Geometry check sheet. Reference: the model listing, model coordinates, mm. A direction names the side the tool comes from. Coordinates: 2 decimals unless noted, no trailing zeros. Order: outer loops, then holes, each group sorted by start corner. A loop starts at its lowest first (then second) coordinate and runs counter-clockwise, first axis right, second up. Notation, with made-up numbers: (-21.5, 58) - (1.5, 58) arc R28 cw to (1.5, 97) - close; hole circle Ø5 at (-11.5, 17.5). An arc over 180 degrees is marked (long way). Put each result on its own line as item: value.
from build123d import *

# Parameters (mm, degrees)
CROQUIS1_W                         = 500
CROQUIS1_H                         = 510
SALIENTE_EXTRUIR1_DEPTH            = 6.35
CORTAR_EXTRUIR1_DEPTH              = 358.16287951
CORTAR_EXTRUIR2_DEPTH              = 358.16287951
TALADRO_ROSCADO_M6X1_01_AT_2_COUNT = 2
TALADRO_ROSCADO_M6X1_01_AT_2_PITCH = 44
TALADRO_ROSCADO_M6X1_01_AT_3_COUNT = 2
TALADRO_ROSCADO_M6X1_01_AT_3_PITCH = 71.217975259
TALADRO_ROSCADO_M6X1_01_AT_4_COUNT = 2
TALADRO_ROSCADO_M6X1_01_AT_4_PITCH = 56
MATRIZL1_COUNT                     = 4
MATRIZL1_PITCH                     = 10
TALADRO_ROSCADO_M5X0_82_D          = 4.2
TALADRO_ROSCADO_M6X1_02_D          = 5


with BuildPart() as part:
    # Croquis1 → Saliente-Extruir1 (new body)
    with BuildSketch(Plane.XY):
        Rectangle(CROQUIS1_W, CROQUIS1_H)
    extrude(amount=SALIENTE_EXTRUIR1_DEPTH)

    # Croquis2 → Cortar-Extruir1 (cut, through all)
    with BuildSketch(Plane.XY.offset(6.35)):
        with BuildLine():
            Line((-211, -225.15), (-131, -225.15))
            ThreePointArc((-131, -225.15), (-124.65, -231.5), (-131, -237.85))
            Line((-131, -237.85), (-211, -237.85))
            ThreePointArc((-211, -237.85), (-217.35, -231.5), (-211, -225.15))
        make_face()
        with BuildLine():
            Line((-211, 237.85), (-131, 237.85))
            ThreePointArc((-131, 237.85), (-124.65, 231.5), (-131, 225.15))
            Line((-131, 225.15), (-211, 225.15))
            ThreePointArc((-211, 225.15), (-217.35, 231.5), (-211, 237.85))
        make_face()
        with BuildLine():
            Line((131, 237.85), (211, 237.85))
            ThreePointArc((211, 237.85), (217.35, 231.5), (211, 225.15))
            Line((211, 225.15), (131, 225.15))
            ThreePointArc((131, 225.15), (124.65, 231.5), (131, 237.85))
        make_face()
        with BuildLine():
            Line((131, -225.15), (211, -225.15))
            ThreePointArc((211, -225.15), (217.35, -231.5), (211, -237.85))
            Line((211, -237.85), (131, -237.85))
            ThreePointArc((131, -237.85), (124.65, -231.5), (131, -225.15))
        make_face()
        with BuildLine():
            Line((-14.65, -160.73303664), (-14.65, -182.26696336))
            ThreePointArc((-14.65, -182.26696336), (-21, -184), (-27.35, -182.26696336))
            Line((-27.35, -182.26696336), (-27.35, -160.73303664))
            ThreePointArc((-27.35, -160.73303664), (-21, -159), (-14.65, -160.73303664))
        make_face()
    extrude(amount=-CORTAR_EXTRUIR1_DEPTH, mode=Mode.SUBTRACT)

    # Croquis4 → Cortar-Extruir2 (cut, through all)
    with BuildSketch(Plane.XY.offset(6.35)):
        with BuildLine():
            Line((-150, 130), (150, 130))
            ThreePointArc((150, 130), (175, 105), (150, 80))
            Line((150, 80), (-150, 80))
            ThreePointArc((-150, 80), (-175, 105), (-150, 130))
        make_face()
        with BuildLine():
            Line((-150, -28.46), (150, -28.46))
            ThreePointArc((150, -28.46), (175, -53.46), (150, -78.46))
            Line((150, -78.46), (-150, -78.46))
            ThreePointArc((-150, -78.46), (-175, -53.46), (-150, -28.46))
        make_face()
    extrude(amount=-CORTAR_EXTRUIR2_DEPTH, mode=Mode.SUBTRACT)

    # Croquis7 → Taladro roscado M6x1.01 (revolve, cut)
    with BuildSketch(Plane(origin=(-242, 217, 6.35), x_dir=(0, -1, 0), z_dir=(1, 0, 0))):
        Polygon((0, 0), (0, 18.502151548), (2.5, 17), (2.5, 0), align=None)
    taladro_roscado_m6x1_01 = revolve(axis=Axis((-242, 217, 12.7), (0, 0, -1)), mode=Mode.SUBTRACT)

    # Taladro roscado M6x1.01 at 2: Taladro roscado M6x1.01 ×2
    with Locations(*[(i * TALADRO_ROSCADO_M6X1_01_AT_2_PITCH, 0, 0) for i in range(1, TALADRO_ROSCADO_M6X1_01_AT_2_COUNT)]):
        add(taladro_roscado_m6x1_01, mode=Mode.SUBTRACT)

    # Taladro roscado M6x1.01 at 3: Taladro roscado M6x1.01 ×2
    with Locations(*[Vector(0.6178215519319036, -0.7863183388224226, 0) * (i * TALADRO_ROSCADO_M6X1_01_AT_3_PITCH) for i in range(1, TALADRO_ROSCADO_M6X1_01_AT_3_COUNT)]):
        add(taladro_roscado_m6x1_01, mode=Mode.SUBTRACT)

    # Taladro roscado M6x1.01 at 4: Taladro roscado M6x1.01 ×2
    with Locations(*[(0, -i * TALADRO_ROSCADO_M6X1_01_AT_4_PITCH, 0) for i in range(1, TALADRO_ROSCADO_M6X1_01_AT_4_COUNT)]):
        add(taladro_roscado_m6x1_01, mode=Mode.SUBTRACT)

    # MatrizL1: Taladro roscado M6x1.01 ×4
    with Locations(*[(0, -i * MATRIZL1_PITCH, 0) for i in range(1, MATRIZL1_COUNT)]):
        add(taladro_roscado_m6x1_01, mode=Mode.SUBTRACT)

    # MatrizL1 copy 1 sketch → MatrizL1 copy 1 (revolve, cut)
    with BuildSketch(Plane(origin=(-198, 207, 6.35), x_dir=(0, -1, 0), z_dir=(1, 0, 0))):
        Polygon((0, 0), (0, 18.502151548), (2.5, 17), (2.5, 0), align=None)
    revolve(axis=Axis((-198, 207, 12.7), (0, 0, -1)), mode=Mode.SUBTRACT)

    # MatrizL1 copy 2 sketch → MatrizL1 copy 2 (revolve, cut)
    with BuildSketch(Plane(origin=(-198, 197, 6.35), x_dir=(0, -1, 0), z_dir=(1, 0, 0))):
        Polygon((0, 0), (0, 18.502151548), (2.5, 17), (2.5, 0), align=None)
    revolve(axis=Axis((-198, 197, 12.7), (0, 0, -1)), mode=Mode.SUBTRACT)

    # MatrizL1 copy 3 sketch → MatrizL1 copy 3 (revolve, cut)
    with BuildSketch(Plane(origin=(-198, 187, 6.35), x_dir=(0, -1, 0), z_dir=(1, 0, 0))):
        Polygon((0, 0), (0, 18.502151548), (2.5, 17), (2.5, 0), align=None)
    revolve(axis=Axis((-198, 187, 12.7), (0, 0, -1)), mode=Mode.SUBTRACT)

    # MatrizL1 copy 4 sketch → MatrizL1 copy 4 (revolve, cut)
    with BuildSketch(Plane(origin=(-198, 151, 6.35), x_dir=(0, -1, 0), z_dir=(1, 0, 0))):
        Polygon((0, 0), (0, 18.502151548), (2.5, 17), (2.5, 0), align=None)
    revolve(axis=Axis((-198, 151, 12.7), (0, 0, -1)), mode=Mode.SUBTRACT)

    # MatrizL1 copy 5 sketch → MatrizL1 copy 5 (revolve, cut)
    with BuildSketch(Plane(origin=(-198, 141, 6.35), x_dir=(0, -1, 0), z_dir=(1, 0, 0))):
        Polygon((0, 0), (0, 18.502151548), (2.5, 17), (2.5, 0), align=None)
    revolve(axis=Axis((-198, 141, 12.7), (0, 0, -1)), mode=Mode.SUBTRACT)

    # MatrizL1 copy 6 sketch → MatrizL1 copy 6 (revolve, cut)
    with BuildSketch(Plane(origin=(-198, 131, 6.35), x_dir=(0, -1, 0), z_dir=(1, 0, 0))):
        Polygon((0, 0), (0, 18.502151548), (2.5, 17), (2.5, 0), align=None)
    revolve(axis=Axis((-198, 131, 12.7), (0, 0, -1)), mode=Mode.SUBTRACT)

    # MatrizL1 copy 7 sketch → MatrizL1 copy 7 (revolve, cut)
    with BuildSketch(Plane(origin=(-242, 151, 6.35), x_dir=(0, -1, 0), z_dir=(1, 0, 0))):
        Polygon((0, 0), (0, 18.502151548), (2.5, 17), (2.5, 0), align=None)
    revolve(axis=Axis((-242, 151, 12.7), (0, 0, -1)), mode=Mode.SUBTRACT)

    # MatrizL1 copy 8 sketch → MatrizL1 copy 8 (revolve, cut)
    with BuildSketch(Plane(origin=(-242, 141, 6.35), x_dir=(0, -1, 0), z_dir=(1, 0, 0))):
        Polygon((0, 0), (0, 18.502151548), (2.5, 17), (2.5, 0), align=None)
    revolve(axis=Axis((-242, 141, 12.7), (0, 0, -1)), mode=Mode.SUBTRACT)

    # MatrizL1 copy 9 sketch → MatrizL1 copy 9 (revolve, cut)
    with BuildSketch(Plane(origin=(-242, 131, 6.35), x_dir=(0, -1, 0), z_dir=(1, 0, 0))):
        Polygon((0, 0), (0, 18.502151548), (2.5, 17), (2.5, 0), align=None)
    revolve(axis=Axis((-242, 131, 12.7), (0, 0, -1)), mode=Mode.SUBTRACT)

    # Taladro roscado M5x0.82 (through all)
    with Locations(Plane.XY.offset(6.35)):
        with Locations((-125, 193.27), (-125, 163.27), (25, 193.27), (25, 163.27), (175, 193.27), (175, 163.27), (175, -111.73), (175, -141.73), (25, -111.73), (25, -141.73), (-125, -111.73), (-125, -141.73)):
            Hole(TALADRO_ROSCADO_M5X0_82_D / 2)

    # Taladro roscado M6x1.02 (through all)
    with Locations(Plane.XY.offset(6.35)):
        with Locations((-229.542734314, 48.77), (-216.542734314, 48.77), (-216.542734314, 2.77), (-229.542734314, 2.77)):
            Hole(TALADRO_ROSCADO_M6X1_02_D / 2)


solid = part.part
Q1. Depth check by flat-ended pin: pin 1 Ø4.5 at (x, y) = (-242, 187) entering from +Z. Enter the tip coordinate at first touch or a pass-through.
Answer block:
pin 1: passes through
Q2. Section check C-C on z = 4.75. State how many separate pieces and enclosed holes the cut face has, then the cut area to 3 significant figures.
Answer block:
separate pieces: 1
enclosed holes: 39
area: 216,000 mm^2
Q3. Draft check along X on faces 3 (the cylindrical face through (-174.994, 104.45, 3.219)), 4 (the cylindrical face through (174.994, -52.91, 3.219)), 5 (the flat face through (-3, 4, 6.35)). Enter one of: pulls with the +X half, pulls with the -X half, needs draft (parallel to the pull), parting line crosses it, or undercut.
Answer block:
face 3: undercut
face 4: undercut
face 5: needs draft
Q4. Section check B-B on y = -176.5. Record the boundary of the cut face in (x, z), then the cut area to 3 significant figures.
Answer block:
outline: (-250, 0) - (-27.35, 0) - (-27.35, 6.35) - (-250, 6.35) - close; (-14.65, 0) - (250, 0) - (250, 6.35) - (-14.65, 6.35) - close
area: 3,090 mm^2
Q5. Thickness scan on L1, parallel to Y at x = 43, z = 5.75; L2, parallel to X at y = -141.73, z = 1.75; L3, parallel to Y at x = -208.5, z = 4. Record the ranges inside material, lowest first. Write a range as [from, to].
Answer block:
L1: y = [-255, -78.46], [-28.46, 80], [130, 255]
L2: x = [-250, -127.1], [-122.9, 22.9], [27.1, 172.9], [177.1, 250]
L3: y = [-255, -237.85], [-225.15, 225.15], [237.85, 255]
Q6. Access from +Z, -Z, +X, -X, +Y, -Y to the whole of each face (thin tool, end or side, straight path). Record for faces 1 (the cylindrical face through (-174.994, -54.01, 3.219)), 2 (the flat face through (-3, 4, 0)).
Answer block:
face 1: +Z, -Z
face 2: -Z, +X, -X, +Y, -Y
Q7. Section check A-A on x = 183. Record the boundary of the cut face in (y, z), then the cut area to 3 significant figures.
Answer block:
outline: (-255, 0) - (-237.85, 0) - (-237.85, 6.35) - (-255, 6.35) - close; (-225.15, 0) - (225.15, 0) - (225.15, 6.35) - (-225.15, 6.35) - close; (237.85, 0) - (255, 0) - (255, 6.35) - (237.85, 6.35) - close
area: 3,080 mm^2
Q8. Section check D-D on x = 83.5. Record the boundary of the cut face in (y, z), then the cut area to 3 significant figures.
Answer block:
outline: (-255, 0) - (-78.46, 0) - (-78.46, 6.35) - (-255, 6.35) - close; (-28.46, 0) - (80, 0) - (80, 6.35) - (-28.46, 6.35) - close; (130, 0) - (255, 0) - (255, 6.35) - (130, 6.35) - close
area: 2,600 mm^2
